from build123d import *

# Parameters (mm, degrees)
F0_R     = 20
F1_DEPTH = 22
F3_DEPTH = 25
F4_W     = 10
F4_H     = 25


with BuildPart() as f1:
    # F0 (on Front) → F1 (new body)
    with BuildSketch(Plane.XZ):
        Circle(F0_R)
    extrude(amount=F1_DEPTH)

    # F2 (on face) → F3 (join)
    with BuildSketch(Plane.XZ.offset(22)):
        Polygon((6.8819096024, -5), (6.8819096024, 5), (-2.6286555606, 8.0901699437), (-8.5065080835, 0), (-2.6286555606, -8.0901699437), align=None)
    extrude(amount=F3_DEPTH)

    # F4 (on face) → F5 (revolve)
    with BuildSketch(Plane(origin=(2.1266270209, 0, 6.5450849719), x_dir=(0.9510565163, 0, -0.3090169944), z_dir=(0.3090169944, 0, 0.9510565163))):
        with Locations((0, -34.5)):
            Rectangle(F4_W, F4_H)
    revolve(axis=Axis((-2.6286555606, -34.5, 8.0901699437), (0, -1, 0)))


solid = f1.part
Here's how the part is built. I have some questions about the finished solid (model axes, mm). A direction names the side the tool comes from. Give positions to 0.01 mm unless a question says otherwise; leave off trailing zeros. Order: outer loops, then holes, each group sorted by start corner. A loop starts at its lowest first (then second) coordinate and runs counter-clockwise, first axis right, second up. Notation, with made-up numbers: (-39.75, 59.5) -> (13.25, 59.5) arc R27 ccw to (13.25, 83.5) -> close; hole circle Ø10 at (67, 88). An arc over 180 degrees is marked (long way). One line per item, written item: value. Start each with the question number.
1. Imagine slicing it at D-D, the plane x = 10.5. List the corners of the cut face in (y, z) for me, plus the area to 3 significant figures.
2. Imagine slicing it at B-B, the plane y = -11.5. List the corners of the cut face in (x, z) for me.
3. Will these pins go through, and if not, where does the flat tip stop? pin 1 Ø2 at (x, y) = (3, -28.5) entering from +Z; pin 2 Ø5 at (y, z) = (-32, 0) entering from +X; pin 3 Ø5 at (x, y) = (12, -20) entering from +Z.
4. For faces 1 (the face through (-5.4, -34.3, 17.7)), 2 (the face through (-4.336, -10.846, -19.524)), 3 (the face through (0, 0, 0)), 4 (the face through (6.882, -34, 0)), 5 (the face through (-5.6, -34.3, -4)), which set-ups out of +Z, -Z, +X, -X, +Y, -Y let a thin tool reach every point of the face, with its end or its side?
5. Imagine slicing it at A-A, the plane x = -7.5. List the corners of the cut face in (y, z) for me, plus the area to 3 significant figures.
6. Imagine slicing it at C-C, the plane z = 2. List the corners of the cut face in (x, y) for me.
7. I need wall thicknesses on probe 1 along Y at (x, z) = (-11, -7.5); probe 2 along X at (y, z) = (-6.5, -6); probe 3 along Z at (x, y) = (4, -38). Which ranges of each line are inside material? Lowest first, please. Write a range as from..to.
Values follow:
1. outline: (-22, -17.02) -> (0, -17.02) -> (0, 17.02) -> (-22, 17.02) -> close
1. area: 749 mm2
2. outline: circle Ø40 at (0, 0)
3. pin 1: stops at z = 16.95
3. pin 2: stops at x = 6.88
3. pin 3: stops at z = 17.6
4. face 1: -Y
4. face 2: +Y, -Y
4. face 3: +Z, -Z, +X, -X, +Y
4. face 4: -Z, +X, -Y
4. face 5: -Z, -X, -Y
5. outline: (-47, -1.39) -> (-22, -1.39) -> (-22, -18.54) -> (0, -18.54) -> (0, 18.54) -> (-22, 18.54) -> (-22, 16.82) -> (-47, 16.82) -> close
5. area: 1,270 mm2
6. outline: (-19.9, -22) -> (-10.56, -22) -> (-10.56, -47) -> (6.88, -47) -> (6.88, -22) -> (19.9, -22) -> (19.9, 0) -> (-19.9, 0) -> close
7. probe 1: y = -22..0
7. probe 2: x = -19.08..19.08
7. probe 3: z = -5.94..15.58
